from build123d import *

# Parameters (mm, degrees)
F1_DEPTH = 191.008
F3_DEPTH = 45.3146


with BuildPart() as f1:
    # F0 (on Right) → F1 (new body)
    with BuildSketch(Plane.YZ):
        with BuildLine():
            ThreePointArc((2.168026, 50.428026), (0.783992, 50.703327), (0, 49.53))
            Line((0, 49.53), (2.168026, 50.428026))
        make_face()
        Polygon((2.168026, 50.428026), (0, 49.53), (0, 3.175), (-18.161, 3.175), (-18.161, 0), (3.175, 0), (3.175, 46.779451), (5.8166, 46.779451), align=None)
        Polygon((-18.161, 0), (-18.161, 3.175), (-36.322, 3.175), (-36.322, 49.53), (-38.490026, 50.428026), (-42.1386, 46.779451), (-39.497, 46.779451), (-39.497, 0), align=None)
        with BuildLine():
            Line((-38.490026, 50.428026), (-36.322, 49.53))
            ThreePointArc((-36.322, 49.53), (-37.105992, 50.703327), (-38.490026, 50.428026))
        make_face()
    extrude(amount=F1_DEPTH)

    # F2 (on face) → F3 (intersect, through all)
    with BuildSketch(Plane(origin=(0, 3.175, 0), x_dir=(-1, 0, 0), z_dir=(0, 1, 0))):
        with BuildLine():
            Line((-26.416, 0), (0, 0))
            Line((0, 0), (0, 4.465561))
            ThreePointArc((0, 4.465561), (-1.508444, 5.628635), (-2.079805, 7.44569))
            Line((-2.079805, 7.44569), (-2.079805, 46.779451))
            ThreePointArc((-2.079805, 46.779451), (-1.508444, 48.596507), (0, 49.759581))
            Line((0, 49.759581), (0, 50.428026))
            Line((0, 50.428026), (-12.231331, 50.428026))
            Line((-12.231331, 50.428026), (-12.231331, 49.759581))
            ThreePointArc((-12.231331, 49.759581), (-9.31908, 49.38309), (-7.961135, 46.779451))
            Line((-7.961135, 46.779451), (-7.961135, 7.44569))
            ThreePointArc((-7.961135, 7.44569), (-9.31908, 4.842052), (-12.231331, 4.465561))
            Line((-12.231331, 4.465561), (-12.231331, 3.797116))
            Line((-12.231331, 3.797116), (-13.247331, 3.797116))
            Line((-13.247331, 3.797116), (-13.247331, 4.465561))
            ThreePointArc((-13.247331, 4.465561), (-16.159581, 4.842052), (-17.517526, 7.44569))
            Line((-17.517526, 7.44569), (-17.517526, 46.779451))
            ThreePointArc((-17.517526, 46.779451), (-16.159581, 49.38309), (-13.247331, 49.759581))
            Line((-13.247331, 49.759581), (-13.247331, 50.428026))
            Line((-13.247331, 50.428026), (-26.416, 50.428026))
            Line((-26.416, 50.428026), (-26.416, 49.759581))
            ThreePointArc((-26.416, 49.759581), (-23.503749, 49.38309), (-22.145805, 46.779451))
            Line((-22.145805, 46.779451), (-22.145805, 7.44569))
            ThreePointArc((-22.145805, 7.44569), (-23.503749, 4.842052), (-26.416, 4.465561))
            Line((-26.416, 4.465561), (-26.416, 0))
        make_face()
    extrude(amount=-F3_DEPTH, mode=Mode.INTERSECT)


solid = f1.part
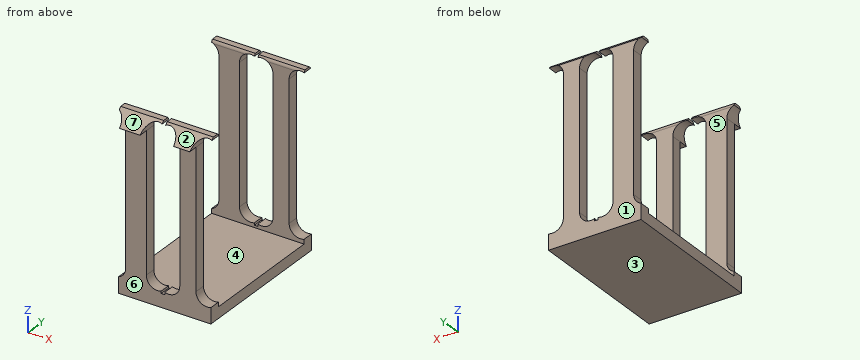
Can you work these out from the model? Positions are in its coordinate system, mm. Face numbers are marked on the shaded views. A direction names the side the tool comes from. Coordinates: 2 decimals unless noted, no trailing zeros. Loops run counter-clockwise (first coordinate to the right, second up) from the corner with the lowest first, then second, coordinate; pieces in that order, holes last. Notation, with made-up numbers: M -27.5,-13.75 L -2.5,-13.75 A24 ccw -2.5,7.25 Z; hole C 56,-19.5 d4. An arc over 180 degrees is marked long. Return JSON: item names as keys, results as strings. Group by question number.
Item 1: Imagine slicing it at B-B (x = 24.5). Please give me the cut outline in (y, z) (3 decimals), and give its area (3 significant figures).
Item 2: Imagine slicing it at A-A (z = 21). Please give me the cut outline in (x, y) (3 decimals), and give its area (3 significant figures).
Item 3: Imagine slicing it at D-D (y = -7). Please give me the cut outline in (x, z) (3 decimals), and give its area (3 significant figures).
Item 4: On a 3-axis mill with a long thin cutter (end or side, diameter ignored), from which of +Z, -Z, +X, -X, +Y, -Y can I reach the whole of each face in a straight line? I mean the marked faces 5, 6 and 7. Say none if no direction works.
Item 5: Thinking about a two-plate mould opening in Y: for the marked faces 1, 2, 3 and 4, which applies, released by +Y, released by -Y, zero draft, split by the parting line, or undercut?
Item 6: Imagine slicing it at C-C (x = 20.75). Please give me the cut outline in (y, z) (3 decimals), and give its area (3 significant figures).
Item 7: If I drill on L1, parallel to X at y = 1, z = 36.5; L2, parallel to Y at x = 2.75, z = 31 (3 decimals); L3, parallel to Z at x = 12.75, y = -19.5 (3 decimals), over which ranges is the centre line in solid material (lowest first)? Write a range as from..to.
Item 8: I'm going to push flat-ended pins straight in: pin 1 Ø2 at (x, y) = (4, -41) entering from -Z; pin 2 Ø3.5 at (y, z) = (2.5, 34.5) entering from +X; pin 3 Ø3 at (y, z) = (-36, 37) entering from -X. Where does each tip first touch, or does it pass through?
Verdict:
{
 "1": {"outline": "M -39.497,0 L 3.175,0 L 3.175,4.379 L 0,4.379 L 0,3.175 L -36.322,3.175 L -36.322,4.379 L -39.497,4.379 Z; M -39.072,49.847 L -36.362,49.847 A1.27 ccw -36.694,50.428 L -38.49,50.428 Z; M 0.04,49.847 L 2.75,49.847 L 2.168,50.428 L 0.372,50.428 A1.27 ccw Z", "area": "146 mm^2"},
 "2": {"outline": "M 2.08,-39.497 L 7.961,-39.497 L 7.961,-36.322 L 2.08,-36.322 Z; M 2.08,0 L 7.961,0 L 7.961,3.175 L 2.08,3.175 Z; M 17.518,-39.497 L 22.146,-39.497 L 22.146,-36.322 L 17.518,-36.322 Z; M 17.518,0 L 22.146,0 L 22.146,3.175 L 17.518,3.175 Z", "area": "66.7 mm^2"},
 "3": {"outline": "M 0,0 L 26.416,0 L 26.416,3.175 L 0,3.175 Z", "area": "83.9 mm^2"},
 "4": {"face 5": "+Z, +X, -X", "face 6": "-Z, +X, -X, -Y", "face 7": "+Z, +X, -X, -Y"},
 "5": {"face 1": "released by +Y", "face 2": "released by -Y", "face 3": "zero draft", "face 4": "undercut"},
 "6": {"outline": "M -42.139,46.779 L -39.497,46.779 L -39.497,0 L 3.175,0 L 3.175,49.421 L 2.168,50.428 L 0.372,50.428 A1.27 ccw 0,49.53 L 0,3.175 L -36.322,3.175 L -36.322,49.53 A1.27 ccw -36.694,50.428 L -38.49,50.428 Z", "area": "438 mm^2"},
 "7": {"L1": "x = 2.08..7.96, 17.52..22.15", "L2": "y = -39.497..-36.322, 0..3.175", "L3": "z = 0..3.175"},
 "8": {"pin 1": "stops at z = 46.78", "pin 2": "stops at x = 22.15", "pin 3": "stops at x = 2.08"}
}
